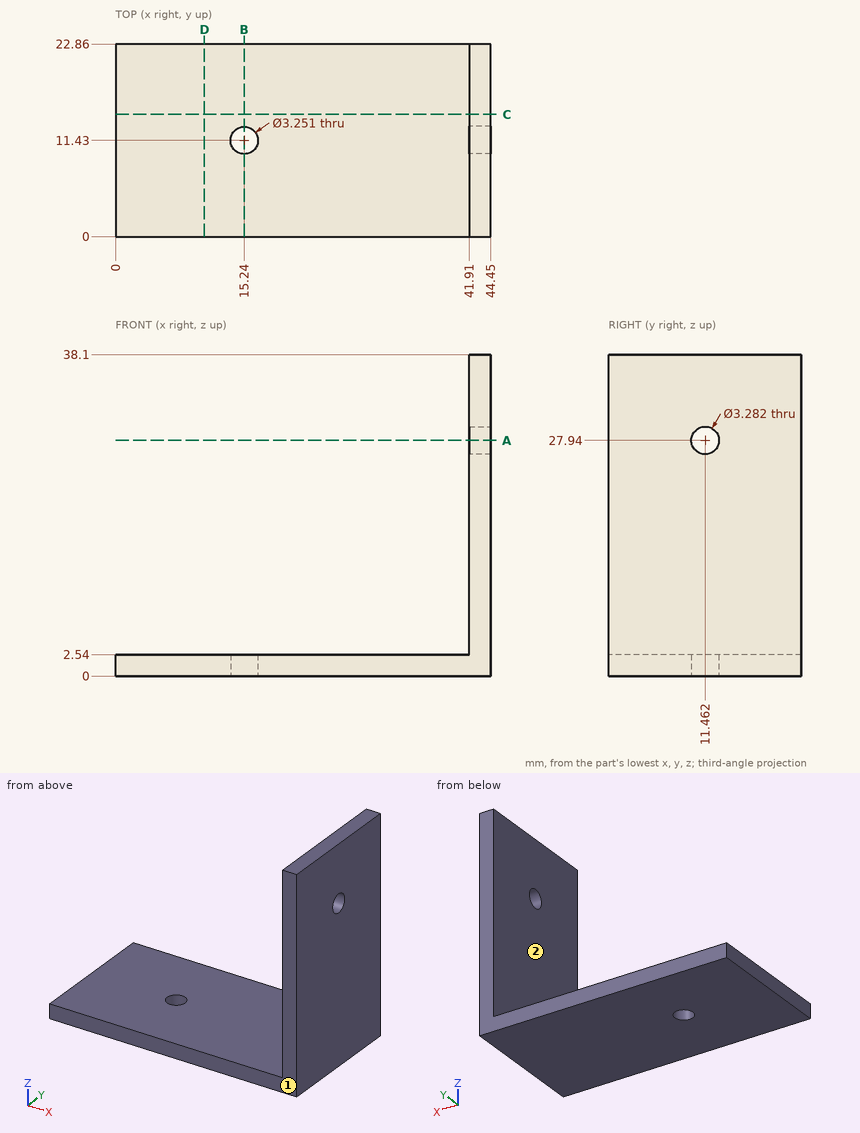
Verification items for this drawing (mm, ordinates from the low corner). A direction names the side the tool comes from. Give positions to 0.01 mm unless a question says otherwise; leave off trailing zeros. Loops run counter-clockwise (first coordinate to the right, second up) from the corner with the lowest first, then second, coordinate; pieces in that order, holes last. Notation, with made-up numbers: M -40,31.25 L -32,31.25 A23 ccw -32,53.25 Z; hole C 82,8 d11. An arc over 180 degrees is marked long. Answer in a Markdown table with one row per item.
1) Depth check by flat-ended pin: pin 1 (4 mm diameter, centred on x = 15.24, y = 11.43, fed in from +Z); pin 2 (10 mm diameter, centred on y = 14, z = 16, fed in from -X). Enter the tip coordinate at first touch or a pass-through.
Solutions:
| item | result |
|---|---|
| pin 1 | stops at z = 2.54 |
| pin 2 | stops at x = 41.91 |
2) Tool access check on the marked faces 1 and 2. Record the directions out of +Z, -Z, +X, -X, +Y, -Y that give a thin tool (end or side, any length) a straight path to the whole face; none if there is none.
Solutions:
| item | result |
|---|---|
| face 1 | +Z, -Z, +X, -X, -Y |
| face 2 | +Z, -X, +Y, -Y |
3) Cross-section at C-C (y = 14.5). Enter the section's corners in (x, z).
Solutions:
| item | result |
|---|---|
| outline | M 0,0 L 44.45,0 L 44.45,38.1 L 41.91,38.1 L 41.91,2.54 L 0,2.54 Z |
4) Thickness scan on line 1 (Y direction, x = 15.24, z = 1.6) (1 decimal); line 2 (Z direction, x = 3, y = 4.25); line 3 (X direction, y = 16, z = 5). Record the ranges inside material, lowest first.
Solutions:
| item | result |
|---|---|
| line 1 | y = 0 to 9.8, 13.1 to 22.9 |
| line 2 | z = 0 to 2.54 |
| line 3 | x = 41.91 to 44.45 |
5) Cross-section at B-B (x = 15.24). Enter the section's corners in (y, z) (1 decimal), plus the area to 3 significant figures.
Solutions:
| item | result |
|---|---|
| outline | M 0,0 L 9.8,0 L 9.8,2.5 L 0,2.5 Z; M 13.1,0 L 22.9,0 L 22.9,2.5 L 13.1,2.5 Z |
| area | 49.8 mm^2 |
6) Cross-section at A-A (z = 27.94). Enter the section's corners in (x, y).
Solutions:
| item | result |
|---|---|
| outline | M 41.91,0 L 44.45,0 L 44.45,9.82 L 41.91,9.82 Z; M 41.91,13.1 L 44.45,13.1 L 44.45,22.86 L 41.91,22.86 Z |
7) Cross-section at D-D (x = 10.5). Enter the section's corners in (y, z).
Solutions:
| item | result |
|---|---|
| outline | M 0,0 L 22.86,0 L 22.86,2.54 L 0,2.54 Z |
